The listing builds one solid part. Answer for the finished solid, in the listing's coordinates (mm). A direction names the side the tool comes from. Give positions to 0.01 mm unless a question says otherwise; leave off trailing zeros. Write each loop counter-clockwise with the first axis right and the second up, starting at its lowest first coordinate (ties: lowest second). Pieces come first, ordered by that corner, then holes. Notation, with made-up numbers: (11, 39.25) - (17, 39.25) arc R18 ccw to (17, 69.25) - close; hole circle Ø3 at (42.5, -14). An arc over 180 degrees is marked (long way). Answer as CSV lines item,"result". Start each with the question number.
(1) Each of these flat-tipped pins is pushed along its axis until it touches: pin 1 Ø16.5 at (x, z) = (110.5, 182.5) entering from +Y; pin 2 Ø4 at (x, z) = (-35, 164) entering from -Y (3 decimals); pin 3 Ø8 at (x, z) = (-80.5, 28.5) entering from +Y. Where does it stop, or does it pass through?
(2) Find section A-A (z = 203.2). State how many separate pieces and enclosed holes the cut face has, then the cut area to 3 significant figures.
(3) For a pull along X with two mould halves and no side action, classify faces 6 (the face through (-99.7, 57.3, 35.3)), 7 (the face through (-104.55, 67.94, 252.19)), 8 (the face through (103, 44.45, 193)), 9 (the face through (125.09, 36.89, 252.19)) as pulls with the +X half, pulls with the -X half, needs draft (parallel to the pull), parting line crosses it, or undercut.
(4) Straight lines are drawn through the part: probe 1 along X at (y, z) = (23, 50); probe 2 along Z at (x, y) = (95, 8.5); probe 3 along X at (y, z) = (22, 50). For each, find the intervals that lie inside material, in ascending order.
(5) For faces 1 (the face through (71.8, 87.7, 252.2)), 2 (the face through (-73.195, 89.122, 128.689)), 3 (the face through (-110.449, 57.35, 189.116)), 4 (the face through (-104.55, 67.94, 1.81)), 5 (the face through (-1, 73.025, 125)), determine the directions among +Z, -Z, +X, -X, +Y, -Y from which every point of the face is accessible in a straight line to the end or side of a thin tool.
(6) Find section B-B (y = 39.5). Write down the section's boundary in (x, z).
(7) Find section C-C (x = -8). Write down the section's boundary in (y, z) (3 decimals), then the cut area to 3 significant figures.
from build123d import *

# Parameters (mm, degrees)
BASE_EXTRUDE_DEPTH                               = 254
CUT_EXTRUDE3_DEPTH                               = 255
FILLET1_R                                        = 6.35
CBORE_FOR_3_4_SOCKET_HEAD_CAP_SCREW1_D           = 19.84248
CBORE_FOR_3_4_SOCKET_HEAD_CAP_SCREW1_CBORE_D     = 31.75
CBORE_FOR_3_4_SOCKET_HEAD_CAP_SCREW1_CBORE_DEPTH = 63.5


with BuildPart() as part:
    # Sketch1 → Base-Extrude (new body)
    with BuildSketch(Plane.XY):
        Polygon((-38.494829198, 73.025), (38.494829198, 73.025), (78.822745501, 3.175), (127, 3.175), (127, 107.95), (-127, 107.95), (-127, 3.175), (-78.822745501, 3.175), align=None)
    extrude(amount=BASE_EXTRUDE_DEPTH)

    # Sketch4 → Cut-Extrude3 (cut, through all)
    with BuildSketch(Plane.XY.offset(254)):
        Polygon((-127, 69.85), (-127, 107.95), (-62.324961559, 107.95), (-84.322006815, 69.85), align=None)
    cut_extrude3 = extrude(amount=-CUT_EXTRUDE3_DEPTH, mode=Mode.SUBTRACT)

    # Mirror1: Cut-Extrude3 across plane
    add(cut_extrude3.mirror(Plane(origin=(0, 0, 0), x_dir=(0, 0, 1), z_dir=(1, 0, 0))), mode=Mode.SUBTRACT)

    # Fillet1
    fillet1_edges = [part.edges().sort_by_distance(p)[0] for p in [
        (127, 36.5125, 0),
        (102.911372751, 3.175, 0),
        (-127, 36.5125, 254),
        (-127, 3.175, 127),
        (127, 3.175, 127),
        (-102.911372751, 3.175, 254),
        (-73.323484187, 88.9, 254),
        (-62.324961559, 107.95, 127),
        (-105.661003408, 69.85, 254),
        (-84.322006815, 69.85, 127),
        (-127, 69.85, 127),
        (-73.323484187, 88.9, 0),
        (-105.661003408, 69.85, 0),
        (0, 107.95, 0),
        (0, 107.95, 254),
        (102.911372751, 3.175, 254),
        (62.324961559, 107.95, 127),
        (105.661003408, 69.85, 0),
        (127, 69.85, 127),
        (73.323484187, 88.9, 0),
        (84.322006815, 69.85, 127),
        (73.323484187, 88.9, 254),
        (105.661003408, 69.85, 254),
        (127, 36.5125, 254),
        (-102.911372751, 3.175, 0),
        (-127, 36.5125, 0),
    ]]
    fillet(fillet1_edges, radius=FILLET1_R)

    # CBORE for 3/4 Socket Head Cap Screw1 (through all)
    with Locations(Plane(origin=(32.15140412, 107.95, 73.186569829), x_dir=(-1, 0, 0), z_dir=(0, 1, 0))):
        with Locations((135.27540412, 130.013430171), (135.27540412, -22.386569829), (-70.97259588, -22.386569829), (-70.97259588, 130.013430171)):
            CounterBoreHole(CBORE_FOR_3_4_SOCKET_HEAD_CAP_SCREW1_D / 2, CBORE_FOR_3_4_SOCKET_HEAD_CAP_SCREW1_CBORE_D / 2, CBORE_FOR_3_4_SOCKET_HEAD_CAP_SCREW1_CBORE_DEPTH)


solid = part.part
Result set:
1,pin 1,"y = 69.85"
1,pin 2,"y = 73.025"
1,pin 3,"y = 83.4"
2,separate pieces,"3"
2,enclosed holes,"0"
2,area,"11,000 mm^2"
3,face 6,"undercut"
3,face 7,"needs draft"
3,face 8,"undercut"
3,face 9,"pulls with the +X half"
4,probe 1,"-127 to -113.01, -93.24 to -67.38, 67.38 to 93.24, 113.01 to 127"
4,probe 2,"0.08 to 45.11, 56.49 to 197.51, 208.89 to 253.92"
4,probe 3,"-127 to -113.01, -93.24 to -67.95, 67.95 to 93.24, 113.01 to 127"
5,face 1,"+Z, +X, +Y"
5,face 2,"+Z, -Z, -X, +Y"
5,face 3,"+Y"
5,face 4,"-Z, -X, +Y"
5,face 5,"+Z, -Z, -Y"
6,outline,"(-127, 6.35) arc R6.35 ccw to (-120.65, 0) - (-57.85, 0) - (-57.85, 254) - (-120.65, 254) arc R6.35 ccw to (-127, 247.65) - close; (57.85, 0) - (120.65, 0) arc R6.35 ccw to (127, 6.35) - (127, 247.65) arc R6.35 ccw to (120.65, 254) - (57.85, 254) - close; hole circle Ø19.84 at (-103.12, 50.8); hole circle Ø19.84 at (-103.12, 203.2); hole circle Ø19.84 at (103.12, 50.8); hole circle Ø19.84 at (103.12, 203.2)"
7,outline,"(73.025, 0) - (101.6, 0) arc R6.35 ccw to (107.95, 6.35) - (107.95, 247.65) arc R6.35 ccw to (101.6, 254) - (73.025, 254) - close"
7,area,"8,850 mm^2"
